Could you check a few things on this model? Use its own coordinates, in mm. A direction names the side the tool comes from. Give positions to 0.01 mm unless a question says otherwise; leave off trailing zeros. Write each loop counter-clockwise with the first axis right and the second up, starting at its lowest first coordinate (ties: lowest second). Pieces come first, ordered by that corner, then holes. Notation, with made-up numbers: (-13, 26) - (-8, 26) arc R20 ccw to (-8, 36) - close; hole circle Ø8 at (9.5, 71.25). An arc over 180 degrees is marked (long way). Answer as a JSON object with one key per item and string values. Group by question number.
```python
from build123d import *

# Parameters (mm, degrees)
F0_W     = 20
F0_H     = 80
F1_DEPTH = 75
F2_W     = 100
F2_H     = 20
F2_R     = 5
F3_DEPTH = 20.001
F5_DEPTH = 25


with BuildPart() as f1:
    # F0 (on Front) → F1 (new body, symmetric)
    with BuildSketch(Plane.XZ):
        Polygon((75, -25), (75, 25), (-25, 25), (-75, 25), (-75, -25), align=None)
        Polygon((-25, 25), (75, 25), (75, 75), (55, 75), (-25, 75), align=None)
        with Locations((65, 115)):
            Rectangle(F0_W, F0_H)
    extrude(amount=F1_DEPTH, both=True)

    # F2 (on face) → F3 (cut, through all)
    with BuildSketch(Plane(origin=(55, 0, 0), x_dir=(0, -1, 0), z_dir=(-1, 0, 0))):
        with Locations((0, 115)):
            Rectangle(F2_W, F2_H)
        with Locations((0, 140)):
            Circle(F2_R)
    extrude(amount=-F3_DEPTH, mode=Mode.SUBTRACT)

    # F4 (on face) → F5 (cut)
    with BuildSketch(Plane.XY.offset(25)):
        with BuildLine():
            Line((-40, -40), (-40, 40))
            ThreePointArc((-40, 40), (-42.928932, 47.071068), (-50, 50))
            ThreePointArc((-50, 50), (-57.071068, 47.071068), (-60, 40))
            Line((-60, 40), (-60, -40))
            ThreePointArc((-60, -40), (-57.071068, -47.071068), (-50, -50))
            ThreePointArc((-50, -50), (-42.928932, -47.071068), (-40, -40))
        make_face()
    extrude(amount=-F5_DEPTH, mode=Mode.SUBTRACT)


solid = f1.part
```
(1) I want a section at A-A, the plane z = 140. Please give me the cut outline in (x, y), and give its area (3 significant figures).
(2) If we mould it in two halves opening along X, with no side actions, what happens to faces 1 (the flat face through (-25, -1, 50)), 2 (the flat face through (65, 50, 115)), 3 (the flat face through (-60, 1, 13))? For each: +X half, -X half, draft (parallel to the pull), parting line (faces both ways), or undercut.
(3) I want a section at D-D, the plane y = 47. Please give me the cut outline in (x, z).
(4) I need wall thicknesses on L1, parallel to Z at x = 66.25, y = 0; L2, parallel to X at y = -9.5, z = 2.5; L3, parallel to X at y = 32, z = 139. Which ranges of each line are inside material? Lowest first, please.
(5) For faces 4 (the flat face through (-40, -1, 13)), 5 (the flat face through (65, -1, 155)), 6 (the flat face through (-61, -1, 25)), 7 (the flat face through (65, 1, 105)), 8 (the flat face through (-75, -1, 0)), which set-ups out of +Z, -Z, +X, -X, +Y, -Y let a thin tool reach every point of the face, with its end or its side?
(6) I want a section at C-C, the plane x = 62. Please give me the cut outline in (y, z), and give its area (3 significant figures).
(7) Will these pins go through, and if not, where does the flat tip stop? P1, Ø12, axis at x = 10, z = 86.5, coming from the -Y side; P2, Ø13, axis at y = 0, z = 140, coming from the -X side; P3, Ø6, axis at x = -47.5, y = -9.5, coming from the +Z side; P4, Ø25, axis at x = -42.5, y = 9.5, coming from the +Z side.
(8) I want a section at B-B, the plane y = 0. Please give me the cut outline in (x, z), and give its area (3 significant figures).
Entries:
{
 "1": {"outline": "(55, -75) - (75, -75) - (75, -5) - (55, -5) - close; (55, 5) - (75, 5) - (75, 75) - (55, 75) - close", "area": "2,800 mm^2"},
 "2": {"face 1": "-X half", "face 2": "draft", "face 3": "undercut"},
 "3": {"outline": "(-75, -25) - (75, -25) - (75, 105) - (55, 105) - (55, 75) - (-25, 75) - (-25, 25) - (-42.86, 25) - (-42.86, 0) - (-57.14, 0) - (-57.14, 25) - (-75, 25) - close; (55, 125) - (75, 125) - (75, 155) - (55, 155) - close"},
 "4": {"L1": "-25 to 105, 125 to 135, 145 to 155", "L2": "-75 to -60, -40 to 75", "L3": "55 to 75"},
 "5": {"face 4": "+Z", "face 5": "+Z, +X, -X, +Y, -Y", "face 6": "+Z, -X, +Y, -Y", "face 7": "+X, -X", "face 8": "+Z, -Z, -X, +Y, -Y"},
 "6": {"outline": "(-75, -25) - (75, -25) - (75, 155) - (-75, 155) - close; hole (-50, 105) - (50, 105) - (50, 125) - (-50, 125) - close; hole circle Ø10 at (0, 140)", "area": "24,900 mm^2"},
 "7": {"P1": "through", "P2": "x = 55", "P3": "z = 0", "P4": "z = 25"},
 "8": {"outline": "(-75, -25) - (75, -25) - (75, 105) - (55, 105) - (55, 75) - (-25, 75) - (-25, 25) - (-40, 25) - (-40, 0) - (-60, 0) - (-60, 25) - (-75, 25) - close; (55, 125) - (75, 125) - (75, 135) - (55, 135) - close; (55, 145) - (75, 145) - (75, 155) - (55, 155) - close", "area": "13,000 mm^2"}
}
